Build history of the part. All positions in model axes, mm. A direction names the side the tool comes from. Coordinates: 2 decimals unless noted, no trailing zeros. Write each loop counter-clockwise with the first axis right and the second up, starting at its lowest first coordinate (ties: lowest second). Pieces come first, ordered by that corner, then holes.
from build123d import *

# Parameters (mm, degrees)
F1_W         = 7.5
F1_H         = 3
F2_DEPTH     = 14
F0_W         = 7.5
F0_H         = 16
F0_R         = 2.75
F3_DEPTH     = 3
F4_R         = 1.65
F5_DEPTH     = 25
F6_T1_DEPTH  = 11.5
F6_T3_DEPTH  = 5.9
F6_T5_DEPTH  = 18.2
F6_T7_DEPTH  = 17.2
F6_T9_DEPTH  = 15
F6_T11_DEPTH = 16
F6_S15_W     = 0.8
F6_S15_H     = 0.8
F6_T16_DEPTH = 0.8
F6_S21_W     = 0.8
F6_S21_H     = 0.8
F6_T22_DEPTH = 0.8
F6_T37_DEPTH = 18
F6_T41_DEPTH = 17
F6_T48_DEPTH = 18
F6_T52_DEPTH = 17


# Not quite as in the source:
# - a fillet or chamfer that OpenCascade refuses, or shapes differently, is made with other operations: its cross-section is extruded or revolved along the edge and cut away or added


with BuildPart() as f2:
    # F1 (on face) → F2 (new body)
    with BuildSketch(Plane.XY):
        with Locations((3.75, 14.5)):
            Rectangle(F1_W, F1_H)
    extrude(amount=F2_DEPTH)

    # F0 (on Top) → F3 (join)
    with BuildSketch(Plane.XY):
        with Locations((3.75, 8)):
            Rectangle(F0_W, F0_H)
        with Locations((3.75, 8)):
            Circle(F0_R, mode=Mode.SUBTRACT)
    extrude(amount=-F3_DEPTH)

    # F4 (on face) → F5 (cut)
    with BuildSketch(Plane(origin=(0, 16, 0), x_dir=(-1, 0, 0), z_dir=(0, 1, 0))):
        with Locations((-4, 3.4267012961)):
            Circle(F4_R)
        with Locations((-4, 10.6111699715)):
            Circle(F4_R)
    extrude(amount=-F5_DEPTH, mode=Mode.SUBTRACT)

    # F6: fillet of radius 0.8 on 17 edges, made by hand

    # F6_s2 → F6_t1 (cut)
    with BuildSketch(Plane.YZ.offset(-2)):
        with BuildLine():
            ThreePointArc((16, 13.2), (15.7656854249, 13.7656854249), (15.2, 14))
            Line((15.2, 14), (16, 14))
            Line((16, 14), (16, 13.2))
        make_face()
        with BuildLine():
            ThreePointArc((13.8, 14), (13.2343145751, 13.7656854249), (13, 13.2))
            Line((13, 13.2), (13, 14))
            Line((13, 14), (13.8, 14))
        make_face()
        with BuildLine():
            ThreePointArc((0.8, 0), (0.2343145751, -0.2343145751), (0, -0.8))
            Line((0, -0.8), (0, 0))
            Line((0, 0), (0.8, 0))
        make_face()
        with BuildLine():
            ThreePointArc((0, -2.2), (0.2343145751, -2.7656854249), (0.8, -3))
            Line((0.8, -3), (0, -3))
            Line((0, -3), (0, -2.2))
        make_face()
    extrude(amount=F6_T1_DEPTH, mode=Mode.SUBTRACT)

    # F6_s4 → F6_t3 (cut)
    with BuildSketch(Plane.YZ.offset(0.8)):
        with BuildLine():
            ThreePointArc((16, -2.2), (15.7656854249, -2.7656854249), (15.2, -3))
            Line((15.2, -3), (16, -3))
            Line((16, -3), (16, -2.2))
        make_face()
    extrude(amount=F6_T3_DEPTH, mode=Mode.SUBTRACT)

    # F6_s6 → F6_t5 (cut)
    with BuildSketch(Plane.XY.offset(-2.2)):
        with BuildLine():
            ThreePointArc((0, 15.2), (0.2343145751, 15.7656854249), (0.8, 16))
            Line((0.8, 16), (0, 16))
            Line((0, 16), (0, 15.2))
        make_face()
        with BuildLine():
            ThreePointArc((6.7, 16), (7.2656854249, 15.7656854249), (7.5, 15.2))
            Line((7.5, 15.2), (7.5, 16))
            Line((7.5, 16), (6.7, 16))
        make_face()
    extrude(amount=F6_T5_DEPTH, mode=Mode.SUBTRACT)

    # F6_s8 → F6_t7 (cut)
    with BuildSketch(Plane.XZ.offset(-15.2)):
        with BuildLine():
            ThreePointArc((0, -2.2), (0.2343145751, -2.7656854249), (0.8, -3))
            Line((0.8, -3), (0, -3))
            Line((0, -3), (0, -2.2))
        make_face()
        with BuildLine():
            ThreePointArc((6.7, -3), (7.2656854249, -2.7656854249), (7.5, -2.2))
            Line((7.5, -2.2), (7.5, -3))
            Line((7.5, -3), (6.7, -3))
        make_face()
    extrude(amount=F6_T7_DEPTH, mode=Mode.SUBTRACT)

    # F6_s10 → F6_t9 (cut)
    with BuildSketch(Plane.XZ.offset(-13)):
        with BuildLine():
            ThreePointArc((0, -0.8), (0.2343145751, -0.2343145751), (0.8, 0))
            Line((0.8, 0), (0, 0))
            Line((0, 0), (0, -0.8))
        make_face()
        with BuildLine():
            ThreePointArc((6.7, 0), (7.2656854249, -0.2343145751), (7.5, -0.8))
            Line((7.5, -0.8), (7.5, 0))
            Line((7.5, 0), (6.7, 0))
        make_face()
    extrude(amount=F6_T9_DEPTH, mode=Mode.SUBTRACT)

    # F6_s12 → F6_t11 (cut)
    with BuildSketch(Plane.XY):
        with BuildLine():
            ThreePointArc((0, 13.8), (0.2343145751, 13.2343145751), (0.8, 13))
            Line((0.8, 13), (0, 13))
            Line((0, 13), (0, 13.8))
        make_face()
        with BuildLine():
            ThreePointArc((6.7, 13), (7.2656854249, 13.2343145751), (7.5, 13.8))
            Line((7.5, 13.8), (7.5, 13))
            Line((7.5, 13), (6.7, 13))
        make_face()
    extrude(amount=F6_T11_DEPTH, mode=Mode.SUBTRACT)


with BuildPart() as f6_tool14:
    # F6_s15 → F6_t16 (new body)
    with BuildSketch(Plane.XZ.offset(-15.2)):
        with Locations((7.1, -2.6)):
            Rectangle(F6_S15_W, F6_S15_H)
    extrude(amount=-F6_T16_DEPTH)

    # F6_s17 → F6_t18 (revolve, cut)
    with BuildSketch(Plane(origin=(6.7, 15.2, -2.2), x_dir=(-0.7071067812, 0, 0.7071067812), z_dir=(-0.7071067812, 0, -0.7071067812))):
        with BuildLine():
            ThreePointArc((0, -0.8), (0.8, 0), (0, 0.8))
            Line((0, 0.8), (0, -0.8))
        make_face()
    revolve(axis=Axis((6.7, 15.2, -2.2), (0, 1, 0)), mode=Mode.SUBTRACT)


with BuildPart() as f2_1:
    add(f2.part)

    # F6_t13: cut F6_tool14
    add(f6_tool14.part, mode=Mode.SUBTRACT)


with BuildPart() as f6_tool20:
    # F6_s21 → F6_t22 (new body)
    with BuildSketch(Plane.YZ.offset(0.8)):
        with Locations((15.6, -2.6)):
            Rectangle(F6_S21_W, F6_S21_H)
    extrude(amount=-F6_T22_DEPTH)

    # F6_s23 → F6_t24 (revolve, cut)
    with BuildSketch(Plane(origin=(0.8, 15.2, -2.2), x_dir=(0, -0.7071067812, 0.7071067812), z_dir=(0, -0.7071067812, -0.7071067812))):
        with BuildLine():
            ThreePointArc((0, -0.8), (0.8, 0), (0, 0.8))
            Line((0, 0.8), (0, -0.8))
        make_face()
    revolve(axis=Axis((0.8, 15.2, -2.2), (-1, 0, 0)), mode=Mode.SUBTRACT)


with BuildPart() as f2_2:
    add(f2_1.part)

    # F6_t19: cut F6_tool20
    add(f6_tool20.part, mode=Mode.SUBTRACT)

    # F6_s25 → F6_t26 (revolve, cut)
    with BuildSketch(Plane.XY.offset(10.6111699715)):
        with BuildLine():
            ThreePointArc((1.55, 16), (2.1156854249, 15.7656854249), (2.35, 15.2))
            Line((2.35, 15.2), (2.35, 16))
            Line((2.35, 16), (1.55, 16))
        make_face()
    revolve(axis=Axis((4, 16, 10.6111699715), (0, 1, 0)), mode=Mode.SUBTRACT)

    # F6_s27 → F6_t28 (revolve, cut)
    with BuildSketch(Plane.XY.offset(3.4267012961)):
        with BuildLine():
            ThreePointArc((1.55, 16), (2.1156854249, 15.7656854249), (2.35, 15.2))
            Line((2.35, 15.2), (2.35, 16))
            Line((2.35, 16), (1.55, 16))
        make_face()
    revolve(axis=Axis((4, 16, 3.4267012961), (0, 1, 0)), mode=Mode.SUBTRACT)

    # F6_s29 → F6_t30 (revolve, cut)
    with BuildSketch(Plane.XZ.offset(-8)):
        with BuildLine():
            ThreePointArc((7.3, -3), (6.7343145751, -2.7656854249), (6.5, -2.2))
            Line((6.5, -2.2), (6.5, -3))
            Line((6.5, -3), (7.3, -3))
        make_face()
    revolve(axis=Axis((3.75, 8, -3), (0, 0, 1)), mode=Mode.SUBTRACT)

    # F6_s31 → F6_t32 (revolve, cut)
    with BuildSketch(Plane.XZ.offset(-8)):
        with BuildLine():
            ThreePointArc((7.3, 0), (6.7343145751, -0.2343145751), (6.5, -0.8))
            Line((6.5, -0.8), (6.5, 0))
            Line((6.5, 0), (7.3, 0))
        make_face()
    revolve(axis=Axis((3.75, 8, 0), (0, 0, 1)), mode=Mode.SUBTRACT)


with BuildPart() as f6_tool35:
    # F6_s36 → F6_t37 (new body)
    with BuildSketch(Plane.XY.offset(-2)):
        with BuildLine():
            ThreePointArc((0, 13.8), (0.2343145751, 13.2343145751), (0.8, 13))
            Line((0.8, 13), (0, 13))
            Line((0, 13), (0, 13.8))
        make_face()
    extrude(amount=F6_T37_DEPTH)

    split(bisect_by=Plane.XY, keep=Keep.BOTTOM)


with BuildPart() as f6_tool39:
    # F6_s40 → F6_t41 (new body)
    with BuildSketch(Plane.XZ.offset(-15)):
        with BuildLine():
            ThreePointArc((0, -0.8), (0.2343145751, -0.2343145751), (0.8, 0))
            Line((0.8, 0), (0, 0))
            Line((0, 0), (0, -0.8))
        make_face()
    extrude(amount=F6_T41_DEPTH)

    split(bisect_by=Plane.XZ.offset(-13), keep=Keep.BOTTOM)


with BuildPart() as f6_tool35_1:
    add(f6_tool35.part)

    # F6_t43: intersect F6_tool39
    add(f6_tool39.part, mode=Mode.INTERSECT)


with BuildPart() as f2_3:
    add(f2_2.part)

    # F6_t33: cut F6_tool35
    add(f6_tool35_1.part, mode=Mode.SUBTRACT)


with BuildPart() as f6_tool46:
    # F6_s47 → F6_t48 (new body)
    with BuildSketch(Plane.XY.offset(-2)):
        with BuildLine():
            ThreePointArc((6.7, 13), (7.2656854249, 13.2343145751), (7.5, 13.8))
            Line((7.5, 13.8), (7.5, 13))
            Line((7.5, 13), (6.7, 13))
        make_face()
    extrude(amount=F6_T48_DEPTH)

    split(bisect_by=Plane.XY, keep=Keep.BOTTOM)


with BuildPart() as f6_tool50:
    # F6_s51 → F6_t52 (new body)
    with BuildSketch(Plane.XZ.offset(2)):
        with BuildLine():
            ThreePointArc((6.7, 0), (7.2656854249, -0.2343145751), (7.5, -0.8))
            Line((7.5, -0.8), (7.5, 0))
            Line((7.5, 0), (6.7, 0))
        make_face()
    extrude(amount=-F6_T52_DEPTH)

    split(bisect_by=Plane.XZ.offset(-13), keep=Keep.BOTTOM)


with BuildPart() as f6_tool46_1:
    add(f6_tool46.part)

    # F6_t54: intersect F6_tool50
    add(f6_tool50.part, mode=Mode.INTERSECT)


with BuildPart() as f2_4:
    add(f2_3.part)

    # F6_t44: cut F6_tool46
    add(f6_tool46_1.part, mode=Mode.SUBTRACT)


solid = f2_4.part
(1) Slice it at C-C, the plane y = 8. List the corners of the cut face in (x, z).
(2) 3-axis set-ups, long thin cutter, end or side, ignore diameter. For faces 1 (the flat face through (4, 15, 14)), 2 (the cylindrical face through (0.23, 7.71, -2.76)), 3 (the flat face through (4, 13, 7)), 4 (the cylindrical face through (7.26, 7, -0.23)), 5 (the cylindrical face through (0.23, 7, -0.24)): which of +Z, -Z, +X, -X, +Y, -Y reach the whole face in a straight line?
(3) Slice it at B-B, the plane z = 7. List the corners of the cut face in (x, y), and give its area (3 significant figures).
(4) Flat gauge pins, fed straight in: P1, Ø1.5, axis at x = 4, z = 5, coming from the -Y side; P2, Ø1.5, axis at x = 2.5, y = 12, coming from the +Z side. Where does each tip first touch, or does it go through?
(5) Probe L1, parallel to Z at x = 4, y = 14.2; L2, parallel to X at y = 13.75, z = 6.25; L3, parallel to Z at x = 6.5, y = 11.75. List the from-to ranges inside material, lowest first.
(6) Slice it at D-D, the plane x = 4.5. Give the number of separate pieces and of enclosed holes in the cut face, and give its area (3 significant figures).
(7) Slice it at A-A, the plane y = 2.75. List the corners of the cut face in (x, z), and give its area (3 significant figures).
(8) Two-plate mould, pull along X, no slides. Class faces 6 (the cylindrical face through (7.26, 13.23, 6.5)), 7 (the cylindrical face through (5.31, 14.12, 9.61)), 8 (the cylindrical face through (5.65, 14.12, 3.5)), 9 (the flat face through (4, 3, -3)): pulls with the +X half, pulls with the -X half, needs draft (parallel to the pull), parting line crosses it, or undercut.
Results:
1. outline: (0, -2.2) arc R0.8 ccw to (0.5, -2.94) arc R0.8 ccw to (1, -2.2) - (1, -0.8) arc R0.8 ccw to (0.5, -0.06) arc R0.8 ccw to (0, -0.8) - close; (6.5, -2.2) arc R0.8 ccw to (7, -2.94) arc R0.8 ccw to (7.5, -2.2) - (7.5, -0.8) arc R0.8 ccw to (7, -0.06) arc R0.8 ccw to (6.5, -0.8) - close
2. face 1: +Z, +X, -X, +Y, -Y
2. face 2: -Z, -X, +Y, -Y
2. face 3: +Z, +X, -X, -Y
2. face 4: +Z, +X, -Y
2. face 5: +Z, -X, -Y
3. outline: (0, 13.8) arc R0.8 ccw to (0.8, 13) - (6.7, 13) arc R0.8 ccw to (7.5, 13.8) - (7.5, 15.2) arc R0.8 ccw to (6.7, 16) - (0.8, 16) arc R0.8 ccw to (0, 15.2) - close
3. area: 22.0 mm2
4. P1: stops at y = 13
4. P2: stops at z = 0
5. L1: z = -3 to 1.78, 5.08 to 8.96, 12.26 to 14
5. L2: x = 0 to 7.5
5. L3: z = -3 to 0
6. separate pieces: 4
6. enclosed holes: 0
6. area: 53.4 mm2
7. outline: (0, -2.2) arc R0.8 ccw to (0.8, -3) - (6.7, -3) arc R0.8 ccw to (7.5, -2.2) - (7.5, -0.8) arc R0.8 ccw to (6.7, 0) - (0.8, 0) arc R0.8 ccw to (0, -0.8) - close
7. area: 22.0 mm2
8. face 6: pulls with the +X half
8. face 7: undercut
8. face 8: undercut
8. face 9: needs draft
